Autodesk Inventor part; units mm, degrees
ref_plane "YZ Plane" through (0, 0, 0) normal (1, 0, 0) x (0, 1, 0)
ref_plane "XZ Plane" through (0, 0, 0) normal (0, 1, 0) x (-1, 0, 0)
ref_plane "XY Plane" through (0, 0, 0) normal (0, 0, 1) x (1, 0, 0)
sketch "스케치1" plane through (0, 0, 0) normal (0, 0, 1) x (1, 0, 0)
  line L0 (-16.9, 16.9) -> (16.9, 16.9)
  line L1 (16.9, 16.9) -> (16.9, -16.9)
  line L2 (16.9, -16.9) -> (-16.9, -16.9)
  line L3 (-16.9, -16.9) -> (-16.9, 16.9)
  point P0 (0, 0)
  dimension "d0" = 33.8
  dimension "d1" = 33.8
  dimension "d2" = 16.9
  dimension "d3" = 16.9
extrude "돌출1" add sketch "스케치1" along normal blind 3
sketch "스케치2" plane through (0, 0, 3) normal (0, 0, 1) x (1, 0, 0)
  circle A0 centre (-14, 14) radius 1.25
  circle A1 centre (14, 14) radius 1.25
  circle A2 centre (-14, -14) radius 1.25
  circle A3 centre (14, -14) radius 1.25
  line L0 (-16.9, 16.9) -> (-16.9, -16.9)
  line L1 (16.9, 16.9) -> (-16.9, 16.9)
  line L2 (16.9, -16.9) -> (16.9, 16.9)
  line L3 (-16.9, -16.9) -> (16.9, -16.9)
  line L4 (-16.9, 16.9) -> (-11.1, 16.9)
  line L5 (-11.1, 16.9) -> (-11.1, 11.1)
  line L6 (-11.1, 11.1) -> (-16.9, 11.1)
  line L7 (-16.9, 11.1) -> (-16.9, 16.9)
  line L8 (16.9, 16.9) -> (11.1, 16.9)
  line L9 (11.1, 16.9) -> (11.1, 11.1)
  line L10 (11.1, 11.1) -> (16.9, 11.1)
  line L11 (16.9, 11.1) -> (16.9, 16.9)
  line L12 (-16.9, -16.9) -> (-11.1, -16.9)
  line L13 (-11.1, -16.9) -> (-11.1, -11.1)
  line L14 (-11.1, -11.1) -> (-16.9, -11.1)
  line L15 (-16.9, -11.1) -> (-16.9, -16.9)
  line L16 (16.9, -16.9) -> (11.1, -16.9)
  line L17 (11.1, -16.9) -> (11.1, -11.1)
  line L18 (11.1, -11.1) -> (16.9, -11.1)
  line L19 (16.9, -11.1) -> (16.9, -16.9)
  point P0 (0, 0)
  dimension "d6" = 2.5
  dimension "d7" = 2.5
  dimension "d8" = 2.5
  dimension "d9" = 2.5
  dimension "d10" = 2.9
  dimension "d11" = 2.9
  dimension "d12" = 2.9
  dimension "d13" = 2.9
  dimension "d14" = 2.9
  dimension "d15" = 2.9
  dimension "d16" = 2.9
  dimension "d17" = 2.9
  dimension "d18" = 5.8
  dimension "d19" = 5.8
  dimension "d20" = 11.1
  dimension "d21" = 5.8
  dimension "d22" = 5.8
  dimension "d23" = 5.8
  dimension "d24" = 5.8
  dimension "d25" = 5.8
  dimension "d26" = 5.8
extrude "돌출2" add sketch "스케치2" along normal blind 2 contours A0 | A1 | A2 | A3 | L1 L5 L6 L0 | L14 L13 L3 L0 | L1 L2 L10 L9 | L17 L18 L2 L3
sketch "스케치3" plane through (0, 0, 5) normal (0, 0, 1) x (1, 0, 0)
  circle A0 centre (-14, 14) radius 1.5
  circle A1 centre (14, 14) radius 1.5
  circle A2 centre (14, -14) radius 1.5
  circle A3 centre (-14, -14) radius 1.5
  line L0 (-16.9, -11.1) -> (-16.9, -16.9)
  line L1 (-16.9, -16.9) -> (-11.1, -16.9)
  line L2 (11.1, -16.9) -> (16.9, -16.9)
  line L3 (16.9, -16.9) -> (16.9, -11.1)
  line L4 (11.1, 11.1) -> (16.9, 11.1)
  line L5 (16.9, 11.1) -> (16.9, 16.9)
  line L6 (-16.9, 16.9) -> (-16.9, 11.1)
  line L7 (-11.1, 16.9) -> (-16.9, 16.9)
  point P0 (0, 0)
  dimension "d29" = 3
  dimension "d30" = 3
  dimension "d31" = 3
  dimension "d32" = 3
  dimension "d33" = 2.9
  dimension "d34" = 2.9
  dimension "d35" = 2.9
  dimension "d36" = 2.9
  dimension "d37" = 2.9
  dimension "d38" = 2.9
  dimension "d39" = 2.9
  dimension "d40" = 2.9
extrude "돌출3" cut sketch "스케치3" against normal up to surface (5 mm away)
sketch "스케치4" plane through (0, 0, 3) normal (0, 0, 1) x (1, 0, 0)
  line L0 (-7.5, 7.5) -> (7.5, 7.5)
  line L1 (7.5, 7.5) -> (7.5, -7.5)
  line L2 (7.5, -7.5) -> (-7.5, -7.5)
  line L3 (-7.5, -7.5) -> (-7.5, 7.5)
  point P0 (0, 0)
  dimension "d43" = 15
  dimension "d44" = 15
  dimension "d45" = 7.5
  dimension "d46" = 7.5
extrude "돌출4" cut sketch "스케치4" against normal up to surface (3 mm away)
sketch "스케치5" plane through (0, 0, 3) normal (0, 0, 1) x (1, 0, 0)
  line L0 (-7.5, -2.75) -> (-12, -2.75)
  line L1 (-12, -2.75) -> (-12, 2.75)
  line L2 (-12, 2.75) -> (-7.5, 2.75)
  line L3 (-7.5, 2.75) -> (-7.5, -2.75)
  line L4 (7.5, 2.75) -> (12, 2.75)
  line L5 (12, 2.75) -> (12, -2.75)
  line L6 (12, -2.75) -> (7.5, -2.75)
  line L7 (7.5, -2.75) -> (7.5, 2.75)
  line L8 (-7.5, -7.5) -> (-7.5, 7.5)
  line L9 (7.5, 7.5) -> (7.5, -7.5)
  point P0 (0, 0)
  dimension "d49" = 4.5
  dimension "d50" = 5.5
  dimension "d51" = 4.5
  dimension "d52" = 5.5
  dimension "d53" = 0
  dimension "d54" = 2.75
  dimension "d55" = 0
  dimension "d56" = 2.75
extrude "돌출5" cut sketch "스케치5" against normal up to surface (3 mm away)
fillet "모깎기1" radius 2 4 edges at (-12, 2.75, 1.5) (-12, -2.75, 1.5) (12, -2.75, 1.5) (12, 2.75, 1.5)
sketch "스케치6" plane through (0, 0, 0) normal (0, 0, -1) x (-1, 0, 0)
  line L0 (16.9, 16.9) -> (-16.9, 16.9)
  line L1 (-7, 16.9) -> (7, 16.9)
  line L2 (7, 16.9) -> (7, 12.9)
  line L3 (7, 12.9) -> (-7, 12.9)
  line L4 (-7, 12.9) -> (-7, 16.9)
  line L5 (-7, -16.9) -> (7, -16.9)
  line L6 (7, -16.9) -> (7, -12.9)
  line L7 (7, -12.9) -> (-7, -12.9)
  line L8 (-7, -12.9) -> (-7, -16.9)
  line L9 (-16.9, -16.9) -> (16.9, -16.9)
  point P0 (0, 0)
  dimension "d60" = 4
  dimension "d61" = 4
  dimension "d62" = 4
  dimension "d63" = 14
  dimension "d64" = 7
  dimension "d65" = 7
  dimension "d66" = 14
extrude "돌출6" add sketch "스케치6" along normal blind 6
sketch "스케치7" plane through (-11.1, -16.9, 3) normal (0, -1, 0) x (1, 0, 0)
  circle A0 centre (14.6, -6) radius 1.6
  circle A1 centre (7.6, -6) radius 1.6
  line L0 (18.1, -3) -> (18.1, -9)
  line L1 (4.1, -3) -> (4.1, -9)
  line L2 (18.1, -9) -> (4.1, -9)
  point P0 (11.1, -3)
  dimension "d69" = 3.2
  dimension "d70" = 3.5
  dimension "d71" = 3.5
  dimension "d72" = 3
  dimension "d73" = 3
  dimension "d74" = 3.2
extrude "돌출7" cut sketch "스케치7" against normal up to surface (33.8 mm away)
fillet "모깎기2" radius 4 4 edges at (-7, 14.9, -6) (7, 14.9, -6) (-7, -14.9, -6) (7, -14.9, -6)
fillet "모깎기2" radius 3 4 edges at (-16.9, 16.9, 2.5) (-16.9, -16.9, 2.5) (16.9, 16.9, 2.5) (16.9, -16.9, 2.5)
sketch "스케치10" plane through (0, 0, 0) normal (0, 0, -1) x (-1, 0, 0)
  line L0 (7, -16.9) -> (7, -12.9)
  line L1 (-7.5, -7.5) -> (7.5, -7.5)
  line L2 (7, -12.9) -> (-7, -12.9)
  line L3 (-7, -12.9) -> (-7, -7.5)
  line L4 (-7, -7.5) -> (7, -7.5)
  line L5 (7, -7.5) -> (7, -12.9)
  line L6 (-7, -12.9) -> (-7, -16.9)
  line L7 (-7.5, 7.5) -> (7.5, 7.5)
  line L8 (-7, 12.9) -> (7, 12.9)
  line L9 (7, 12.9) -> (7, 7.5)
  line L10 (7, 7.5) -> (-7, 7.5)
  line L11 (-7, 7.5) -> (-7, 12.9)
  point P0 (0, 0)
  dimension "d94" = 14
  dimension "d96" = 14
  dimension "d99" = 14
extrude "돌출10" cut sketch "스케치10" against normal blind 1
equation "\"d72\" = d73"
equation "\"d96\" = d94"
properties part number "Camera_Cover" material "LCP 플라스틱"
Can you work these out from the model? Positions are in its coordinate system, mm. A direction names the side the tool comes from. Round coordinates to 2 decimals unless told otherwise and drop trailing zeros. Loops run counter-clockwise (first coordinate to the right, second up) from the corner with the lowest first, then second, coordinate; pieces in that order, holes last. Notation, with made-up numbers: (63.5, -19) -> (109.5, -19) arc R4 ccw to (109.5, -14) -> close; hole circle Ø8 at (37.25, -4). An arc over 180 degrees is marked (long way). One line per item, written item: value. Start each with the question number.
1. If we section it at C-C, the plane z = 2: Write out the boundary of the cut face in (x, y).
2. For faces 4 (the flat face through (0, -10, 1)), 5 (the flat face through (-14, 11.1, 4)), 6 (the flat face through (-12.8, 12.8, 5)), 7 (the flat face through (-13, 0, 0)), 8 (the flat face through (-7.5, -5, 2)), which set-ups out of +Z, -Z, +X, -X, +Y, -Y let a thin tool reach every point of the face, with its end or its side?
3. If I drill on probe 1 along Y at (x, z) = (14, 1.7); probe 2 along X at (y, z) = (0, 0.75); probe 3 along Z at (x, y) = (-13.5, -3.5), over which ranges is the centre line in solid material (lowest first)?
4. If we section it at A-A, the plane y = 7: Write out the boundary of the cut face in (x, z), then the cut area to 3 significant figures.
5. If we section it at B-B, the plane z = -0.5: Write out the boundary of the cut face in (x, y), then the cut area to 3 significant figures.
6. For pin 1 (1.6 mm diameter, centred on y = -15.5, z = -1.5, fed in from +X); pin 2 (2 mm diameter, centred on x = -6, y = 6, fed in from +Z); pin 3 (1 mm diameter, centred on x = -7.5, y = -9, fed in from -Z); pin 4 (1.5 mm diameter, centred on y = -3.5, z = 3.5, fed in from -X), each with a flat end and sliding along its axis, tell me the tip position at first contact or that it passes through.
7. If we section it at D-D, the plane x = -3.5: Write out the boundary of the cut face in (y, z), then the cut area to 3 significant figures.
8. If we mould it in two halves opening along Z, with no side actions, what happens to faces 1 (the cylindrical face through (3.15, -14.93, -4.56)), 2 (the cylindrical face through (-15.5, 14.07, 2.54)), 3 (the flat face through (-12.8, -12.7, 5))? For each: pulls with the +Z half, pulls with the -Z half, needs draft (parallel to the pull), parting line crosses it, or undercut.
Calculated:
1. outline: (-16.9, -13.9) arc R3 ccw to (-13.9, -16.9) -> (13.9, -16.9) arc R3 ccw to (16.9, -13.9) -> (16.9, 13.9) arc R3 ccw to (13.9, 16.9) -> (-13.9, 16.9) arc R3 ccw to (-16.9, 13.9) -> close; hole circle Ø3 at (-14, -14); hole circle Ø3 at (-14, 14); hole (-12, -0.75) arc R2 ccw to (-10, -2.75) -> (-7.5, -2.75) -> (-7.5, -7.5) -> (7.5, -7.5) -> (7.5, -2.75) -> (10, -2.75) arc R2 ccw to (12, -0.75) -> (12, 0.75) arc R2 ccw to (10, 2.75) -> (7.5, 2.75) -> (7.5, 7.5) -> (-7.5, 7.5) -> (-7.5, 2.75) -> (-10, 2.75) arc R2 ccw to (-12, 0.75) -> close; hole circle Ø3 at (14, -14); hole circle Ø3 at (14, 14)
2. face 4: -Z
2. face 5: +Z, +X, -X
2. face 6: +Z, +X, -X, +Y, -Y
2. face 7: -Z, -X, +Y, -Y
2. face 8: +Z, -Z
3. probe 1: y = -16.9 to -15.5, -12.5 to 12.5, 15.5 to 16.9
3. probe 2: x = -16.9 to -12, 12 to 16.9
3. probe 3: z = 0 to 3
4. outline: (-16.9, 0) -> (-7.5, 0) -> (-7.5, 3) -> (-16.9, 3) -> close; (7.5, 0) -> (16.9, 0) -> (16.9, 3) -> (7.5, 3) -> close
4. area: 56.4 mm²
5. outline: (-7, -16.9) -> (7, -16.9) -> (7, -12.9) -> (-7, -12.9) -> close; (-7, 12.9) -> (7, 12.9) -> (7, 16.9) -> (-7, 16.9) -> close
5. area: 112 mm²
6. pin 1: stops at x = 7
6. pin 2: passes through
6. pin 3: stops at z = 0
6. pin 4: stops at x = -16.9
7. outline: (-16.9, -5.97) -> (-12.9, -5.97) -> (-12.9, -4.6) -> (-16.9, -4.6) -> close; (-16.9, -1.4) -> (-12.9, -1.4) -> (-12.9, 1) -> (-7.5, 1) -> (-7.5, 3) -> (-16.9, 3) -> close; (7.5, 1) -> (12.9, 1) -> (12.9, -1.4) -> (16.9, -1.4) -> (16.9, 3) -> (7.5, 3) -> close; (12.9, -5.97) -> (16.9, -5.97) -> (16.9, -4.6) -> (12.9, -4.6) -> close
7. area: 67.7 mm²
8. face 1: undercut
8. face 2: needs draft
8. face 3: pulls with the +Z half
